```python
from build123d import *

# Parameters (mm, degrees)
F0_W     = 200
F0_H     = 200
F1_DEPTH = 250
F2_T     = -25
F3_W     = 150
F3_H     = 25.2777785063
F4_DEPTH = 175
F5_R     = 201.014082537
F6_DEPTH = 25


with BuildPart() as f1:
    # F0 (on Top) → F1 (new body)
    with BuildSketch(Plane.XY):
        Rectangle(F0_W, F0_H)
    extrude(amount=-F1_DEPTH)

    # F2
    f2_openings = [f1.faces().sort_by_distance(p)[0] for p in [
        (0, -100, -125),
        (0, 0, 0),
        (0, 0, -250),
    ]]
    offset(amount=F2_T, openings=f2_openings)

    # F3 (on face) → F4 (join)
    with BuildSketch(Plane.XZ.offset(-75)):
        with Locations((0, -120.5015406013)):
            Rectangle(F3_W, F3_H)
    extrude(amount=F4_DEPTH)

    # F5 (on face) → F6 (join)
    with BuildSketch(Plane.XY):
        Circle(F5_R)
        Polygon((-75, -100), (-100, -100), (-100, 100), (100, 100), (100, -100), (75, -100), (75, 75), (-75, 75), align=None, mode=Mode.SUBTRACT)
        Polygon((-100, 100), (-100, -100), (-75, -100), (-75, 75), (75, 75), (75, -100), (100, -100), (100, 100), align=None)
    extrude(amount=F6_DEPTH)


solid = f1.part
```
Check sheet for the modelled part. Datum: model origin and axes. Units: mm. A direction names the side the tool comes from. Give positions to 0.01 mm unless a question says otherwise; leave off trailing zeros. Order: outer loops, then holes, each group sorted by start corner. A loop starts at its lowest first (then second) coordinate and runs counter-clockwise, first axis right, second up. Notation, with made-up numbers: M 0.5,9 L 51.5,9 A17 ccw 51.5,35 Z; hole C 68,59.25 d8. An arc over 180 degrees is marked long. Answer in a Markdown table with one row per item. Add a question column.
Q1. Sectioned sample at C-C, the plane z = -33.5. Record the boundary of the cut face in (x, y).
Q2. Thickness scan on L1, parallel to Z at x = 18, y = 29; L2, parallel to X at y = 44, z = -91; L3, parallel to Y at x = 56.5, z = -149.5. Record the ranges inside material, lowest first.
Q3. Gauge pin test, flat ends, axial feed: pin 1 Ø4 at (y, z) = (-100, -54) entering from +X; pin 2 Ø2 at (x, z) = (37, -164) entering from +Y; pin 3 Ø1.5 at (x, y) = (-11.5, -123.5) entering from -Z. Record the tip position at first contact, or that the pin passes through.
Q4. Access from +Z, -Z, +X, -X, +Y, -Y to the whole of each face (thin tool, end or side, straight path). Record for faces 1 (the flat face through (-3, 3, 0)), 2 (the flat face through (-75, -14, -53)), 3 (the flat face through (-75, -14, -191)), 4 (the flat face through (-100, -1, -123)).
Q5. Sectioned sample at A-A, the plane y = 0. Record the boundary of the cut face in (x, z), and give its area (3 significant figures).
Q6. Sectioned sample at D-D, the plane y = -72. Record the boundary of the cut face in (x, z), and give its area (3 significant figures).
Q7. Sectioned sample at B-B, the plane x = 0. Record the boundary of the cut face in (y, z).
Q8. Release check for a two-part mould opening along Z. For faces 5 (the flat face through (-1, -11, -133.14)), 6 (the flat face through (-1, 75, -191)), 7 (the flat face through (75, -14, -53)) record: released by +Z, released by -Z, zero draft, split by the parting line, or undercut.
Verdict:
| question | item | result |
|---|---|---|
| 1 | outline | M -100,-100 L -75,-100 L -75,75 L 75,75 L 75,-100 L 100,-100 L 100,100 L -100,100 Z |
| 2 | L1 | -133.14 to -107.86, 0 to 25 |
| 2 | L2 | -100 to -75, 75 to 100 |
| 2 | L3 | 75 to 100 |
| 3 | pin 1 | x = 100 |
| 3 | pin 2 | y = 100 |
| 3 | pin 3 | z = 0 |
| 4 | face 1 | none |
| 4 | face 2 | -Y |
| 4 | face 3 | -Z, -Y |
| 4 | face 4 | -Z, -X, +Y, -Y |
| 5 | outline | M -201.01,0 L -100,0 L -100,-250 L -75,-250 L -75,-133.14 L 75,-133.14 L 75,-250 L 100,-250 L 100,0 L 201.01,0 L 201.01,25 L -201.01,25 Z; hole M -75,-107.86 L 75,-107.86 L 75,0 L -75,0 Z |
| 5 | area | 26,300 mm² |
| 6 | outline | M -187.68,0 L -100,0 L -100,-250 L -75,-250 L -75,-133.14 L 75,-133.14 L 75,-250 L 100,-250 L 100,0 L 187.68,0 L 187.68,25 L -187.68,25 Z; hole M -75,-107.86 L 75,-107.86 L 75,0 L -75,0 Z |
| 6 | area | 25,700 mm² |
| 7 | outline | M -201.01,0 L 75,0 L 75,-107.86 L -100,-107.86 L -100,-133.14 L 75,-133.14 L 75,-250 L 100,-250 L 100,0 L 201.01,0 L 201.01,25 L -201.01,25 Z |
| 8 | face 5 | released by -Z |
| 8 | face 6 | zero draft |
| 8 | face 7 | undercut |
